from build123d import *

# Parameters (mm, degrees)
SKETCH1_W           = 76.2
SKETCH1_H           = 41.5
BOSS_EXTRUDE1_DEPTH = 3.175
SKETCH2_W           = 3.175
SKETCH2_H           = 15
BOSS_EXTRUDE2_DEPTH = 3.175
SKETCH4_W           = 30
SKETCH4_H           = 3.175
BOSS_EXTRUDE4_DEPTH = 3.175
SKETCH5_W           = 3.175
SKETCH5_H           = 15
BOSS_EXTRUDE5_DEPTH = 3.175
FILLET1_R           = 1


with BuildPart() as part:
    # Sketch1 → Boss-Extrude1 (new body)
    with BuildSketch(Plane.XY):
        Rectangle(SKETCH1_W, SKETCH1_H)
    extrude(amount=BOSS_EXTRUDE1_DEPTH)

    # Sketch2 → Boss-Extrude2 (add)
    with BuildSketch(Plane(origin=(38.1, 0, 0), x_dir=(0, 0, -1), z_dir=(1, 0, 0))):
        with Locations((-1.5875, 3.75)):
            Rectangle(SKETCH2_W, SKETCH2_H)
    extrude(amount=BOSS_EXTRUDE2_DEPTH)

    # Sketch4 → Boss-Extrude4 (add)
    with BuildSketch(Plane.XZ.offset(20.75)):
        with Locations((0, 1.5875)):
            Rectangle(SKETCH4_W, SKETCH4_H)
    extrude(amount=BOSS_EXTRUDE4_DEPTH)

    # Sketch5 → Boss-Extrude5 (add)
    with BuildSketch(Plane.ZY.offset(38.1)):
        with Locations((1.5875, 3.75)):
            Rectangle(SKETCH5_W, SKETCH5_H)
    extrude(amount=BOSS_EXTRUDE5_DEPTH)

    # Fillet1
    fillet1_edges = [part.edges().sort_by_distance(p)[0] for p in [
        (41.275, -3.75, 1.5875),
        (41.275, 11.25, 1.5875),
        (-15, -23.925, 1.5875),
        (15, -23.925, 1.5875),
        (-41.275, -3.75, 1.5875),
        (-41.275, 11.25, 1.5875),
    ]]
    fillet(fillet1_edges, radius=FILLET1_R)


solid = part.part
Input: part model. Units: mm. Frame: model coordinates. A direction names the side the tool comes from. Round coordinates to 2 decimals unless told otherwise and drop trailing zeros. Order: outer loops, then holes, each group sorted by start corner. A loop starts at its lowest first (then second) coordinate and runs counter-clockwise, first axis right, second up. Notation, with made-up numbers: (-26.75, 84.25) - (3.25, 84.25) arc R28 ccw to (3.25, 111.25) - close; hole circle Ø11 at (56, 32). An arc over 180 degrees is marked (long way). Answer as a JSON object with one key per item and string values. Group by question number.
(1) Pin query (flat end, axial travel): P1, Ø1, axis at y = -14.5, z = 1, coming from the -X side; P2, Ø1.7, axis at x = -39.5, z = 2, coming from the +Y side. Return the tip coordinate at first contact, or that it passes through.
(2) Cut plane B-B (x = 34.5). Return loops of the section in (y, z) (3 decimals).
(3) Cut plane A-A (z = 2.15). Return loops of the section in (x, y) (3 decimals).
(4) Cut plane C-C (y = -17). Return loops of the section in (x, z) (3 decimals).
(5) Reachability of faces 1 (the face through (-38.1, -12, 2)), 2 (the face through (38.1, -12, 2)), 3 (the face through (-39, 11.25, 2)), 4 (the face through (-41.275, 4, 2)), 5 (the face through (38.1, 16, 2)) from +Z, -Z, +X, -X, +Y, -Y: full face, straight path, thin tool, end or side. Return the list, or none.
(6) Material intervals for probe 1 along X at (y, z) = (-15, 1.45); probe 2 along Y at (x, z) = (25.5, 2.45), sorted ascending. Write a range as from..to.
Here are the results:
{
 "1": {"P1": "stops at x = -38.1", "P2": "stops at y = 11.25"},
 "2": {"outline": "(-20.75, 0) - (20.75, 0) - (20.75, 3.175) - (-20.75, 3.175) - close"},
 "3": {"outline": "(-41.275, -2.75) arc R1 ccw to (-40.275, -3.75) - (-38.1, -3.75) - (-38.1, -20.75) - (-15, -20.75) - (-15, -22.925) arc R1 ccw to (-14, -23.925) - (14, -23.925) arc R1 ccw to (15, -22.925) - (15, -20.75) - (38.1, -20.75) - (38.1, -3.75) - (40.275, -3.75) arc R1 ccw to (41.275, -2.75) - (41.275, 10.25) arc R1 ccw to (40.275, 11.25) - (38.1, 11.25) - (38.1, 20.75) - (-38.1, 20.75) - (-38.1, 11.25) - (-40.275, 11.25) arc R1 ccw to (-41.275, 10.25) - close"},
 "4": {"outline": "(-38.1, 0) - (38.1, 0) - (38.1, 3.175) - (-38.1, 3.175) - close"},
 "5": {"face 1": "+Z, -Z, -X, -Y", "face 2": "+Z, -Z, +X, -Y", "face 3": "+Z, -Z, -X, +Y", "face 4": "+Z, -Z, -X, +Y, -Y", "face 5": "+Z, -Z, +X, +Y"},
 "6": {"probe 1": "x = -38.1..38.1", "probe 2": "y = -20.75..20.75"}
}
